Build history of the part. All positions in model axes, mm. Coordinates: 2 decimals unless noted, no trailing zeros. Loops run counter-clockwise (first coordinate to the right, second up) from the corner with the lowest first, then second, coordinate; pieces in that order, holes last.
Item 1: Cut at C-C (z = 14). List the corners of the cut face in (x, y), and give its area (3 significant figures).
Item 2: Drill centre lines: line 1 along X through (y, z) = (0.8, 85.5); line 2 along X through (y, z) = (0.4, 48); line 3 along X through (y, z) = (1.3, 20). Where is each one in solid material? Low to high.
Item 3: Cut at A-A (y = 0.95). Count the separate pieces of the cut face and the enclosed holes in it, and give its area (3 significant figures).
Item 4: Flat gauge pin, fed straight in: pin 1 (2 mm diameter, centred on x = 9.37, z = 47.02, fed in from +Y). Where does the tip first touch, or does it go through?
Item 5: Cut at B-B (z = 90.5). List the corners of the cut face in (x, y).
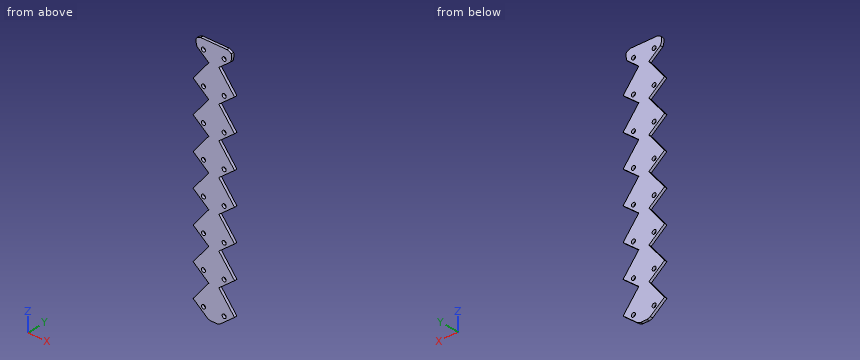
from build123d import *

# Parameters (mm, degrees)
SKETCH2_R           = 1.190625
BOSS_EXTRUDE1_DEPTH = 1.5875
FILLET1_SIZE        = 3.175


with BuildPart() as part:
    # Sketch2 → Boss-Extrude1 (new body)
    with BuildSketch(Plane(origin=(0, 0, 0), x_dir=(1, 0, 0), z_dir=(0, 1, 0))):
        Polygon((-9.038686402, -10.786161972), (0.255627025, -22.394755722), (-9.038686402, -29.836161972), (0.255627025, -41.444755722), (-9.038686402, -48.886161972), (0.255627025, -60.494755722), (-9.038686402, -67.936161972), (0.255627025, -79.544755722), (-9.038686402, -86.986161972), (0.255627025, -98.594755722), (-9.038686402, -106.036161972), (0.255627025, -117.644755722), (-9.038686402, -125.086161972), (-6.062123902, -128.803887343), (12.526502953, -128.803887343), (15.503065453, -125.086161972), (6.208752025, -117.644755722), (15.503065453, -106.036161972), (6.208752025, -98.594755722), (15.503065453, -86.986161972), (6.208752025, -79.544755722), (15.503065453, -67.936161972), (6.208752025, -60.494755722), (15.503065453, -48.886161972), (6.208752025, -41.444755722), (15.503065453, -29.836161972), (6.208752025, -22.394755722), (15.503065453, -10.786161972), (6.208752025, -3.344755722), (15.503065453, 8.263838028), (6.208752025, 15.705244278), (0.255627025, 15.705244278), (-9.038686402, 8.263838028), (0.255627025, -3.344755722), align=None)
        with Locations(Location((-2.903248438, 10.125678468, 0), (0, 0, 270))):
            Circle(SKETCH2_R, mode=Mode.SUBTRACT)
        with Locations(Location((-2.903248438, -8.924321532, 0), (0, 0, 270))):
            Circle(SKETCH2_R, mode=Mode.SUBTRACT)
        with Locations(Location((-2.903248438, -27.974321532, 0), (0, 0, 270))):
            Circle(SKETCH2_R, mode=Mode.SUBTRACT)
        with Locations(Location((-2.903248438, -47.024321532, 0), (0, 0, 270))):
            Circle(SKETCH2_R, mode=Mode.SUBTRACT)
        with Locations(Location((-2.903248438, -66.074321532, 0), (0, 0, 270))):
            Circle(SKETCH2_R, mode=Mode.SUBTRACT)
        with Locations(Location((-2.903248438, -85.124321532, 0), (0, 0, 270))):
            Circle(SKETCH2_R, mode=Mode.SUBTRACT)
        with Locations(Location((-2.903248438, -104.174321532, 0), (0, 0, 270))):
            Circle(SKETCH2_R, mode=Mode.SUBTRACT)
        with Locations(Location((-2.903248438, -123.224321532, 0), (0, 0, 270))):
            Circle(SKETCH2_R, mode=Mode.SUBTRACT)
        with Locations(Location((9.367627489, -123.224321532, 0), (0, 0, 270))):
            Circle(SKETCH2_R, mode=Mode.SUBTRACT)
        with Locations(Location((9.367627489, -104.174321532, 0), (0, 0, 270))):
            Circle(SKETCH2_R, mode=Mode.SUBTRACT)
        with Locations(Location((9.367627489, -85.124321532, 0), (0, 0, 270))):
            Circle(SKETCH2_R, mode=Mode.SUBTRACT)
        with Locations(Location((9.367627489, -66.074321532, 0), (0, 0, 270))):
            Circle(SKETCH2_R, mode=Mode.SUBTRACT)
        with Locations(Location((9.367627489, -47.024321532, 0), (0, 0, 270))):
            Circle(SKETCH2_R, mode=Mode.SUBTRACT)
        with Locations(Location((9.367627489, -27.974321532, 0), (0, 0, 270))):
            Circle(SKETCH2_R, mode=Mode.SUBTRACT)
        with Locations(Location((9.367627489, -8.924321532, 0), (0, 0, 270))):
            Circle(SKETCH2_R, mode=Mode.SUBTRACT)
        with Locations(Location((9.367627489, 10.125678468, 0), (0, 0, 270))):
            Circle(SKETCH2_R, mode=Mode.SUBTRACT)
    extrude(amount=BOSS_EXTRUDE1_DEPTH)

    # Fillet1
    # a fillet whose section is not a circle: 3.175 mm, written as the material it takes off along each edge
    with BuildSketch(Plane(origin=(6.208752025, -2.786065678, -15.705244278), x_dir=(0.7806247497998005, 0, 0.6249999999999992), z_dir=(0, 1, 0)), Plane(origin=(0.255627025, -2.786065678, -15.705244278), x_dir=(1, 0, 0), z_dir=(0, 1, 0))) as fillet1_piece_1:
        with BuildLine():
            Bezier((1.114426271, 0), (0, 0), (-0.869948729, -0.696516419), weights=[1, 0.299581461, 1])
            Line((-0.869948729, -0.696516419), (0, 0))
            Line((0, 0), (1.114426271, 0))
        make_face()
    extrude(amount=7.159631355, mode=Mode.SUBTRACT)
    with BuildSketch(Plane(origin=(-9.038686402, -7.9375, 125.086161972), x_dir=(0.7806247497997997, 0, -0.625), z_dir=(0, 1, 0)), Plane(origin=(15.503065453, -7.9375, 125.086161972), x_dir=(-0.6250000000125396, 0, 0.78062474978976), z_dir=(0, 1, 0))) as fillet1_piece_2:
        with BuildLine():
            Bezier((FILLET1_SIZE, 0), (0, 0), (0, -FILLET1_SIZE), weights=[1, 0.224506403, 1])
            Line((0, -FILLET1_SIZE), (0, 0))
            Line((0, 0), (FILLET1_SIZE, 0))
        make_face()
    extrude(amount=17.4625, mode=Mode.SUBTRACT)
    with BuildSketch(Plane(origin=(12.526502953, -3.813051662, 128.803887343), x_dir=(-1, 0, 0), z_dir=(0, 1, 0)), Plane(origin=(-6.062123902, -3.813051662, 128.803887343), x_dir=(-0.6249999999999978, 0, -0.7806247497998016), z_dir=(0, 1, 0))) as fillet1_piece_3:
        with BuildLine():
            Bezier((1.525220665, 0), (0, 0), (-0.953262916, -1.190625), weights=[1, 0.286190632, 1])
            Line((-0.953262916, -1.190625), (0, 0))
            Line((0, 0), (1.525220665, 0))
        make_face()
    extrude(amount=9.213603325, mode=Mode.SUBTRACT)


solid = part.part
Filled sheet:
1. outline: (-6.47, 0) - (12.93, 0) - (12.93, 1.59) - (-6.47, 1.59) - close
1. area: 30.8 mm2
2. line 1: x = -7.18 to -4.03, -1.77 to 8.24, 10.5 to 13.65
2. line 2: x = -7.93 to -3.59, -2.22 to 8.69, 10.05 to 14.4
2. line 3: x = -1.66 to 8.13
3. separate pieces: 1
3. enclosed holes: 16
3. area: 2,150 mm2
4. pin 1: passes through
5. outline: (-6.23, 0) - (12.69, 0) - (12.69, 1.59) - (-6.23, 1.59) - close
